Check sheet for the modelled part. Datum: model origin and axes. Units: mm. A direction names the side the tool comes from. Round coordinates to 2 decimals unless told otherwise and drop trailing zeros. Order: outer loops, then holes, each group sorted by start corner. A loop starts at its lowest first (then second) coordinate and runs counter-clockwise, first axis right, second up. Notation, with made-up numbers: (19, 30) -> (26, 30) arc R23 ccw to (26, 51) -> close; hole circle Ø7 at (11.25, 3.5). An arc over 180 degrees is marked (long way). Answer in a Markdown table with one row per item. Add a question column.
1. Material ranges on L1, parallel to Y at x = -7.5, z = -7.5; L2, parallel to Y at x = -4, z = -0.25; L3, parallel to Z at x = -10, y = 536, recorded low to high. Write a range as from..to.
2. Depth check by flat-ended pin: P1, Ø3, axis at x = 0, z = 0, coming from the +Y side; P2, Ø12, axis at x = -2.5, y = 483, coming from the -Z side; P3, Ø4.5, axis at x = -2.5, z = -0.5, coming from the -Y side; P4, Ø1, axis at x = 13.5, y = 531, coming from the -Z side. Enter the tip coordinate at first touch or a pass-through.
3. Sectioned sample at C-C, the plane y = 474.5. Record the boundary of the cut face in (x, z), then the cut area to 3 significant figures.
4. Sectioned sample at A-A, the plane y = 414. Record the boundary of the cut face in (x, z).
5. Sectioned sample at B-B, the plane x = 4. Record the boundary of the cut face in (y, z), then the cut area to 3 significant figures.
6. Access from +Z, -Z, +X, -X, +Y, -Y to the whole of each face (thin tool, end or side, straight path). Record for faces 1 (the flat face through (12.578, 412.213, 3.494)), 2 (the flat face through (12.21, 562.28, -3.39)), 3 (the flat face through (-3, 542, -7)).
7. Draft check along Z on faces 4 (the flat face through (-12.578, 412.213, -3.494)), 5 (the flat face through (-11.87, 562.28, -3.49)), 6 (the flat face through (-3, 392, -7)). Enter one of: +Z half, -Z half, draft (parallel to the pull), parting line (faces both ways), or undercut.
8. Sectioned sample at D-D, the plane x = -28. Record the boundary of the cut face in (y, z).
```python
from build123d import *

# Parameters (mm, degrees)
SWEEP_1_DEPTH            = 610
CUT_EXTRUDE_2_DEPTH      = 12
SKETCH_21_R              = 1.75
CUT_EXTRUDE_3_DEPTH      = 600
CUT_EXTRUDE_4_DEPTH      = 691.959477934
CUT_EXTRUDE_4_DEPTH_BACK = 691.959477934
SKETCH_26_OUTSIDE_W      = 208.38
SKETCH_26_OUTSIDE_H      = 816.38
SKETCH_26_OUTSIDE_W_2    = 70
SKETCH_26_OUTSIDE_H_2    = 190
CUT_EXTRUDE_5_DEPTH      = 41
SKETCH_28_OUTSIDE_W      = 112.694
SKETCH_28_OUTSIDE_H      = 62.694
CUT_EXTRUDE_7_DEPTH      = 40


# Read off the part's stored shape, not the designer's step: 扫描1
with BuildPart() as part:
    # 扫描1 outline → 扫描1 (new body)
    with BuildSketch(Plane(origin=(0, 0, 0), x_dir=(1, 0, 0), z_dir=(0, 1, 0))):
        Polygon((-35, 0), (35, 0), (0, 10), align=None)
    sweep_1 = extrude(amount=SWEEP_1_DEPTH)

    # 草图1 → 放样1 section 0
    with BuildSketch(Plane.XY, mode=Mode.PRIVATE) as loft_1_s0:
        with BuildLine():
            Line((-35, 610), (0, 690))
            Line((0, 690), (35, 610))
            Line((35, 610), (-35, 610))
        make_face()
    loft_1 = loft([Vertex(0, 610, -10), loft_1_s0.sketch])

    # 镜向1: 扫描1, 放样1 across plane
    add(sweep_1.mirror(Plane.XY))
    add(loft_1.mirror(Plane.XY))

    # 草图19 → 切除-拉伸2 (cut)
    with BuildSketch(Plane.XZ):
        Polygon((0, -10), (35, 0), (0, 10), (-35, 0), align=None)
    extrude(amount=-CUT_EXTRUDE_2_DEPTH, mode=Mode.SUBTRACT)

    # 草图21 → 切除-拉伸3 (cut)
    with BuildSketch(Plane.XZ.offset(-12)):
        with Locations(Location((0, 0, 0), (0, 0, 270))):
            Circle(SKETCH_21_R)
    extrude(amount=-CUT_EXTRUDE_3_DEPTH, mode=Mode.SUBTRACT)

    # 草图26 outside → 切除-拉伸4 (cut, two sides: drawn at the far end of the back side and taken through both)
    with BuildSketch(Plane.XY.offset(-CUT_EXTRUDE_4_DEPTH_BACK)):
        with Locations((0, 351)):
            Rectangle(SKETCH_26_OUTSIDE_W, SKETCH_26_OUTSIDE_H)
        with Locations((0, 487)):
            Rectangle(SKETCH_26_OUTSIDE_W_2, SKETCH_26_OUTSIDE_H_2, mode=Mode.SUBTRACT)
    extrude(amount=CUT_EXTRUDE_4_DEPTH + CUT_EXTRUDE_4_DEPTH_BACK, mode=Mode.SUBTRACT)

    # 草图27 → 切除-拉伸5 (cut)
    with BuildSketch(Plane.XZ.offset(-392)):
        Polygon((24.807846155, 0), (0, 7.087956044), (-24.807846155, 0), (0, -7.087956044), align=None)
    extrude(amount=-CUT_EXTRUDE_5_DEPTH, mode=Mode.SUBTRACT)

    # 草图28 outside → 切除-拉伸7 (cut)
    with BuildSketch(Plane(origin=(0, 582, 0), x_dir=(1, 0, 0), z_dir=(0, 1, 0))):
        Rectangle(SKETCH_28_OUTSIDE_W, SKETCH_28_OUTSIDE_H)
        Polygon((0, 6.879952905), (-24.079835166, 0), (0, -6.879952905), (24.079835166, 0), align=None, mode=Mode.SUBTRACT)
    extrude(amount=-CUT_EXTRUDE_7_DEPTH, mode=Mode.SUBTRACT)


solid = part.part
```
Answer key:
| question | item | result |
|---|---|---|
| 1 | L1 | y = 392..542 |
| 1 | L2 | y = 433..582 |
| 1 | L3 | z = -7.14..7.14 |
| 2 | P1 | passes through |
| 2 | P2 | stops at z = -10 |
| 2 | P3 | stops at y = 433 |
| 2 | P4 | stops at z = -6.29 |
| 3 | outline | (-35, 0) -> (0, -10) -> (35, 0) -> (0, 10) -> close; hole circle Ø3.5 at (0, 0) |
| 3 | area | 690 mm² |
| 4 | outline | (-35, 0) -> (0, -10) -> (35, 0) -> (0, 10) -> close; hole (-24.81, 0) -> (0, -7.09) -> (24.81, 0) -> (0, 7.09) -> close |
| 5 | outline | (392, -8.86) -> (542, -8.86) -> (542, -5.74) -> (582, -5.74) -> (582, 5.74) -> (542, 5.74) -> (542, 8.86) -> (392, 8.86) -> (392, 5.95) -> (433, 5.95) -> (433, -5.95) -> (392, -5.95) -> close |
| 5 | area | 2,630 mm² |
| 6 | face 1 | -Y |
| 6 | face 2 | -Z, +X, +Y |
| 6 | face 3 | +Y |
| 7 | face 4 | undercut |
| 7 | face 5 | -Z half |
| 7 | face 6 | draft |
| 8 | outline | (392, -2) -> (542, -2) -> (542, 2) -> (392, 2) -> close |
